Geometry: see drawing. Coordinates: mm, zero at the bounding-box minimum. Give positions to 0.01 mm unless a question says otherwise; leave off trailing zeros. Write each loop counter-clockwise with the first axis right and the second up, starting at its lowest first coordinate (ties: lowest second). Pieces come first, ordered by that corner, then holes. Notation, with made-up numbers: (47.25, 57) - (104.25, 57) arc R24 ccw to (104.25, 95) - close; hole circle Ø7 at (57, -28). An arc over 180 degrees is marked (long way). Use a Markdown table: item, result. Add a question column.
1. Material intervals for probe 1 along Z at (x, y) = (7.5, 2.65); probe 2 along X at (y, z) = (0.65, 4) (1 decimal); probe 3 along X at (y, z) = (2.35, 48.5) (1 decimal), sorted ascending.
2. Section query A-A, the plane x = 7.5. Return loops of the section in (y, z), plus the area to 3 significant figures.
3. Section query D-D, the plane z = 36. Return loops of the section in (x, y).
4. Section query B-B, the plane z = 7.5. Return loops of the section in (x, y), plus the area to 3 significant figures.
5. Pin query (flat end, axial travel): pin 1 (3 mm diameter, centred on y = 1, z = 8, fed in from +X); pin 2 (2 mm diameter, centred on x = 37.5, y = 2, fed in from -Z). Return the tip coordinate at first contact, or that it passes through.
6. Section query C-C, the plane y = 0.85. Return loops of the section in (x, z) (1 decimal).
7. Mould query, pull axis X, two halves, no side actions, for the marked faces 1, 2 and 3. Classes: released by +X, released by -X, zero draft, split by the parting line, or undercut.
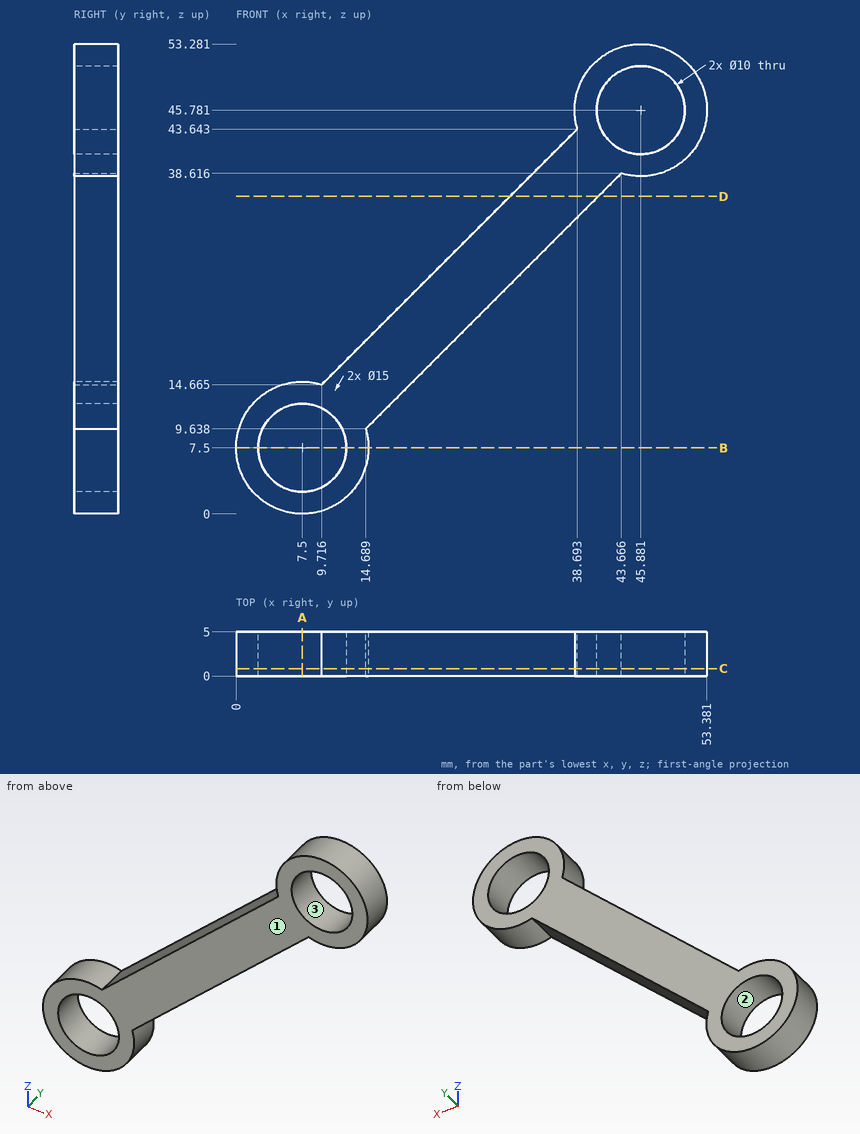
Result sheet:
| question | item | result |
|---|---|---|
| 1 | probe 1 | z = 0 to 2.5, 12.5 to 15 |
| 1 | probe 2 | x = 0.9 to 3.9, 11.1 to 14.1 |
| 1 | probe 3 | x = 38.9 to 41.7, 50.1 to 52.9 |
| 2 | outline | (0, 0) - (5, 0) - (5, 2.5) - (0, 2.5) - close; (0, 12.5) - (5, 12.5) - (5, 15) - (0, 15) - close |
| 2 | area | 25.0 mm² |
| 3 | outline | (31.05, 0) - (41.05, 0) - (41.05, 5) - (31.05, 5) - close |
| 4 | outline | (0, 0) - (2.5, 0) - (2.5, 5) - (0, 5) - close; (12.5, 0) - (15, 0) - (15, 5) - (12.5, 5) - close |
| 4 | area | 25.0 mm² |
| 5 | pin 1 | stops at x = 15 |
| 5 | pin 2 | stops at z = 31.45 |
| 6 | outline | (9.7, 14.7) arc R7.5 ccw (long way) to (14.7, 9.6) - (43.7, 38.6) arc R7.5 ccw (long way) to (38.7, 43.6) - close; hole circle Ø10 at (7.5, 7.5); hole circle Ø10 at (45.9, 45.8) |
| 7 | face 1 | zero draft |
| 7 | face 2 | undercut |
| 7 | face 3 | undercut |
